Check sheet for the drawn part. Datum: minimum x, y, z corner. Units: mm. Round coordinates to 2 decimals unless told otherwise and drop trailing zeros. Write each loop counter-clockwise with the first axis right and the second up, starting at its lowest first coordinate (ties: lowest second). Pieces come first, ordered by that corner, then holes. Notation, with made-up numbers: (-11, -29.75) - (29, -29.75) arc R10 cw to (29, -16.75) - close; hole circle Ø10 at (63, 81). An arc over 180 degrees is marked (long way). Answer as a JSON object with one key per item and string values.
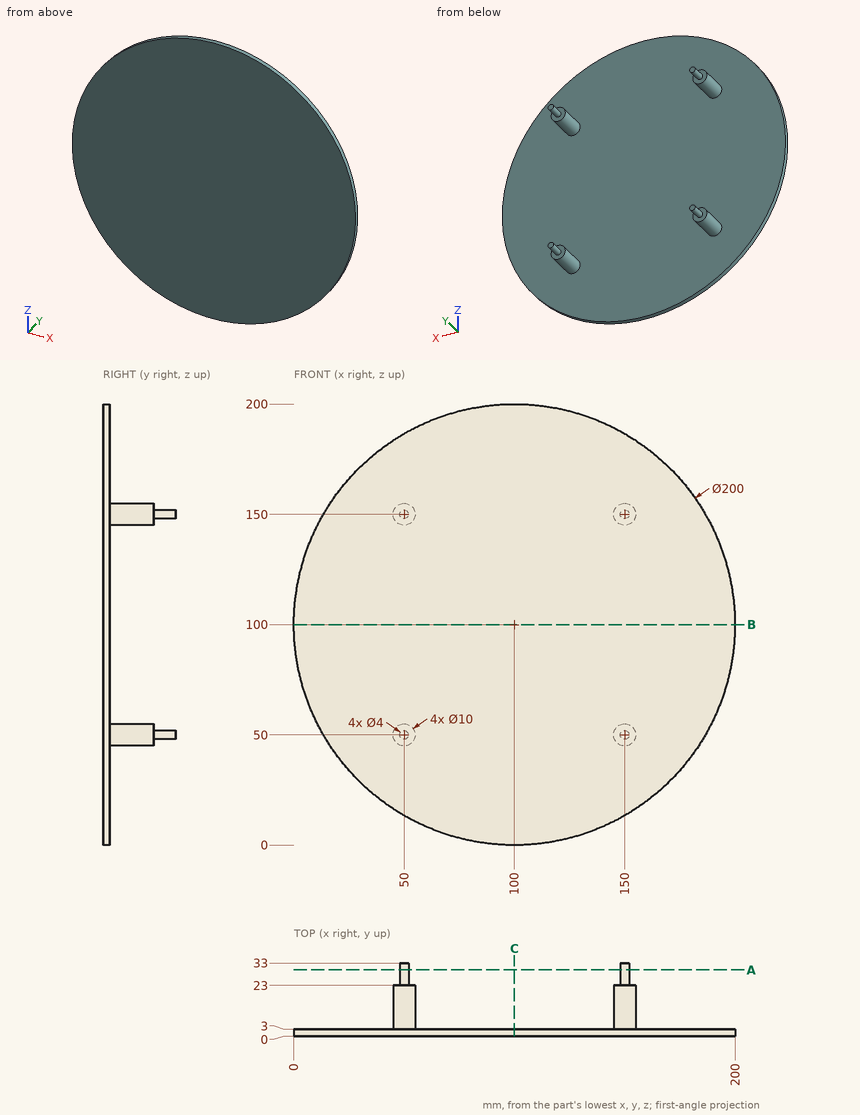
1. Go/stop test with flat-tipped pins: pin 1 (5 mm diameter, centred on x = 48, z = 152.5, fed in from +Y); pin 2 (6 mm diameter, centred on x = 141.5, y = 15.5, fed in from +Z); pin 3 (6 mm diameter, centred on x = 167, z = 122, fed in from +Y). Record where each tip stops, or that it passes through.
Completed:
{"pin 1": "stops at y = 33", "pin 2": "passes through", "pin 3": "stops at y = 3"}
2. Material ranges on probe 1 along Y at (x, z) = (137, 54.5); probe 2 along X at (y, z) = (7.5, 149.5); probe 3 along Z at (x, y) = (153, 16), recorded low to high. Write a range as from..to.
Completed:
{"probe 1": "y = 0..3", "probe 2": "x = 45.03..54.97, 145.03..154.97", "probe 3": "z = 46..54, 146..154"}
3. Cross-section at B-B (z = 100). Record the boundary of the cut face in (x, y).
Completed:
{"outline": "(0, 0) - (200, 0) - (200, 3) - (0, 3) - close"}
4. Cross-section at A-A (y = 30). Record the boundary of the cut face in (x, z).
Completed:
{"outline": "circle Ø4 at (50, 50); circle Ø4 at (50, 150); circle Ø4 at (150, 50); circle Ø4 at (150, 150)"}
5. Cross-section at C-C (x = 100). Record the boundary of the cut face in (y, z).
Completed:
{"outline": "(0, 0) - (3, 0) - (3, 200) - (0, 200) - close"}
